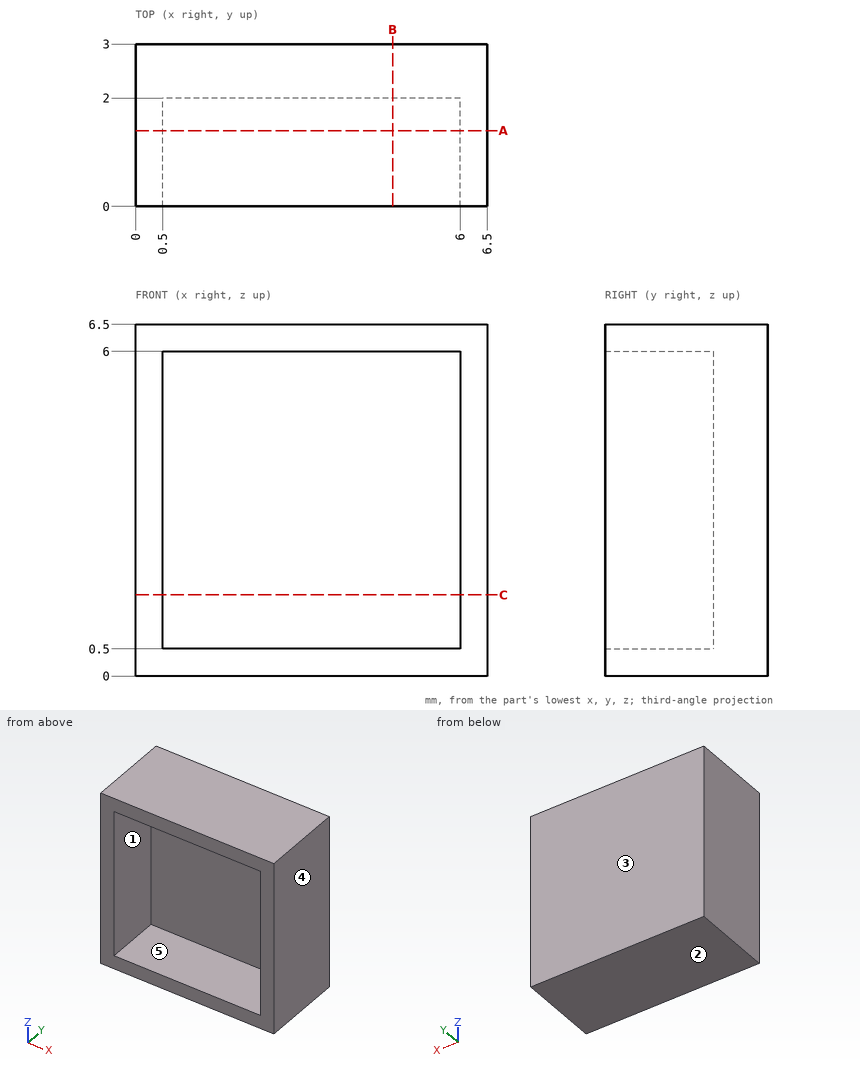
Answer from the drawing. Dimensions are ordinates in mm from the lowest x, y and z of the part. A direction names the side the tool comes from. Give positions to 0.01 mm unless a question says otherwise; leave off trailing zeros. Write each loop counter-clockwise with the first axis right and the second up, starting at its lowest first coordinate (ties: lowest second). Pieces come first, ordered by that corner, then holes. Notation, with made-up numbers: (50, 55) - (88, 55) arc R19 cw to (88, 90) - close; hole circle Ø11 at (-26, 80). An arc over 180 degrees is marked (long way). Answer in a Markdown table with one row per item. Add a question column.
Item 1: A tool of negligible diameter and unlimited length cuts with its end or side. For the marked faces 1 and 2, from which of +Z, -Z, +X, -X, +Y, -Y can it reach the whole face along a straight path? Write none if from no direction.
Item 2: A flat-ended cylindrical pin translates along its axis: P1, Ø1.6, axis at x = 3.5, z = 2.5, coming from the -Y side. Find the tip coordinate at first contact, or state that the pin passes through.
Item 3: Section B-B, the plane x = 4.75 is taken. Write down the section's boundary in (y, z).
Item 4: Determine the mould class of the marked faces 3, 4 and 5 for opening direction X: pulls with the +X half, pulls with the -X half, needs draft (parallel to the pull), parting line crosses it, or undercut.
Item 5: Section A-A, the plane y = 1.4 is taken. Write down the section's boundary in (x, z).
Item 6: Section C-C, the plane z = 1.5 is taken. Write down the section's boundary in (x, y).
Item 7: Find the intervals of material crossed by L1, parallel to X at y = 1.1, z = 1; L2, parallel to Y at x = 5.5, z = 1.75, in increasing order.
Recorded:
| question | item | result |
|---|---|---|
| 1 | face 1 | -Y |
| 1 | face 2 | -Z, +X, -X, +Y, -Y |
| 2 | P1 | stops at y = 2 |
| 3 | outline | (0, 0) - (3, 0) - (3, 6.5) - (0, 6.5) - (0, 6) - (2, 6) - (2, 0.5) - (0, 0.5) - close |
| 4 | face 3 | needs draft |
| 4 | face 4 | pulls with the +X half |
| 4 | face 5 | undercut |
| 5 | outline | (0, 0) - (6.5, 0) - (6.5, 6.5) - (0, 6.5) - close; hole (0.5, 0.5) - (6, 0.5) - (6, 6) - (0.5, 6) - close |
| 6 | outline | (0, 0) - (0.5, 0) - (0.5, 2) - (6, 2) - (6, 0) - (6.5, 0) - (6.5, 3) - (0, 3) - close |
| 7 | L1 | x = 0 to 0.5, 6 to 6.5 |
| 7 | L2 | y = 2 to 3 |
